Input: part model. Units: mm. Frame: model coordinates. A direction names the side the tool comes from. Give positions to 0.01 mm unless a question says otherwise; leave off trailing zeros. Loops run counter-clockwise (first coordinate to the right, second up) from the corner with the lowest first, then second, coordinate; pieces in that order, holes last. Notation, with made-up numbers: (63.5, -33.5) - (120.5, -33.5) arc R31 cw to (120.5, -4.5) - close; hole circle Ø3 at (64.5, 84). An arc over 180 degrees is marked (long way). One line per item, written item: value.
from build123d import *

# Parameters (mm, degrees)
F1_DEPTH = 63.5
F2_DEPTH = 25.4
F3_DEPTH = 7.9375
F0_W     = 25.4
F0_H     = 19.05
F4_DEPTH = 25.4
F6_R     = 5.08


# Not quite as in the source:
# - a feature names something its author has since deleted; it is built from what else it names


with BuildPart() as f1:
    # F0 (on Front) → F1 (new body, symmetric)
    with BuildSketch(Plane.XZ):
        Polygon((22.225, 9.525), (-41.275, 9.525), (-41.275, -9.525), (41.275, -9.525), (41.275, 9.525), align=None)
    extrude(amount=F1_DEPTH, both=True)

    # F0 (on Front) → F2 (join, symmetric)
    with BuildSketch(Plane.XZ):
        with BuildLine():
            Line((22.225, 27.0002), (22.225, 9.525))
            Line((22.225, 9.525), (41.275, 9.525))
            Line((41.275, 9.525), (41.275, 27.0002))
            ThreePointArc((41.275, 27.0002), (45.9246798487, 38.2255201513), (57.15, 42.8752))
            Line((57.15, 42.8752), (60.325, 42.8752))
            Line((60.325, 42.8752), (60.325, 61.9252))
            Line((60.325, 61.9252), (57.15, 61.9252))
            ThreePointArc((57.15, 61.9252), (32.4542956671, 51.6959043329), (22.225, 27.0002))
        make_face()
    extrude(amount=F2_DEPTH, both=True)

    # F0 (on Front) → F3 (join, symmetric)
    with BuildSketch(Plane.XZ):
        with BuildLine():
            add(Edge.make_bspline(
                [(-41.275, 9.525), (-39.190236479, 31.1887320131), (12.7593874931, 62.8514587879), (57.15, 61.9252)],
                knots=[0, 0, 0, 0, 111.5045361635, 111.5045361635, 111.5045361635, 111.5045361635], degree=3))
            Line((-41.275, 9.525), (22.225, 9.525))
            Line((22.225, 9.525), (22.225, 27.0002))
            ThreePointArc((22.225, 27.0002), (32.4542956671, 51.6959043329), (57.15, 61.9252))
        make_face()
    extrude(amount=F3_DEPTH, both=True)

    # F0 (on Front) → F4 (join, symmetric)
    with BuildSketch(Plane.XZ):
        with Locations((73.025, 52.4002)):
            Rectangle(F0_W, F0_H)
    extrude(amount=F4_DEPTH, both=True)

    # F0 (on Front) → F5 (revolve)
    with BuildSketch(Plane.XZ):
        Polygon((85.725, 66.675), (85.725, 61.9252), (85.725, 42.8752), (85.725, 38.1), (111.125, 38.1), (111.125, 66.675), align=None)
    revolve(axis=Axis((85.725, 0, 52.3875), (0, 0, -1)))

    # F6
    f6_edges = [f1.edges().sort_by_distance(p)[0] for p in [
        (41.275, -63.5, 0),
        (-41.275, -63.5, 0),
        (-41.275, 63.5, 0),
        (41.275, 63.5, 0),
    ]]
    fillet(f6_edges, radius=F6_R)


solid = f1.part
Item 1: Access query for faces 4 (the face through (46, -25.4, 42)), 5 (the face through (60, 2, 61.925)), 6 (the face through (45.8, -0.4, 38.1)). Directions: +Z, -Z, +X, -X, +Y, -Y. A direction counts if a zero-diameter tool reaches every point of the face in a straight line with its end or side. Return the directions, or none.
Verdict:
face 4: +Z, +X, -X, -Y
face 5: +Z, -X
face 6: -Z, +Y, -Y
Item 2: Material intervals for L1, parallel to Z at x = 68, y = -18 (3 decimals); L2, parallel to Z at x = -15.5, y = -38.5 (3 decimals); L3, parallel to X at y = -25.5, z = -4 (3 decimals), sorted ascending.
Verdict:
L1: z = 38.1 to 66.675
L2: z = -9.525 to 9.525
L3: x = -41.275 to 41.275
Item 3: Draft query along Y for faces 1 (the face through (1, -36, 9.525)), 2 (the face through (39.8, -62, 0.1)), 3 (the face through (46, 25.4, 42)). Return one class per face: pulls with the +Y half, pulls with the -Y half, needs draft (parallel to the pull), parting line crosses it, or undercut.
Verdict:
face 1: needs draft
face 2: pulls with the -Y half
face 3: pulls with the +Y half
Item 4: Pin query (flat end, axial travel): P1, Ø14, axis at y = 19.5, z = 20, coming from the -X side (3 decimals); P2, Ø8.5, axis at x = 67.5, y = -0.5, coming from the -Z side; P3, Ø4, axis at x = 45, y = -33.5, coming from the +Z side; P4, Ø1, axis at x = 1.5, z = 33, coming from the -Y side. Return the tip coordinate at first contact, or that it passes through.
Verdict:
P1: stops at x = 22.225
P2: stops at z = 38.1
P3: passes through
P4: stops at y = -7.94
Item 5: Section B-B, the plane y = 27.5. Output: boundary loops of the cut face in (x, z) (3 decimals).
Verdict:
outline: (-41.275, -9.525) - (41.275, -9.525) - (41.275, 9.525) - (-41.275, 9.525) - close
Item 6: Section A-A, the plane x = 64. Output: boundary loops of the cut face in (y, z) (3 decimals), and give its area (3 significant figures).
Verdict:
outline: (-25.4, 42.875) - (-13.16, 42.875) - (-13.16, 38.1) - (13.16, 38.1) - (13.16, 42.875) - (25.4, 42.875) - (25.4, 61.925) - (13.16, 61.925) - (13.16, 66.675) - (-13.16, 66.675) - (-13.16, 61.925) - (-25.4, 61.925) - close
area: 1,220 mm^2
Item 7: Section C-C, the plane x = 97. Output: boundary loops of the cut face in (y, z) (3 decimals).
Verdict:
outline: (-22.76, 38.1) - (22.76, 38.1) - (22.76, 66.675) - (-22.76, 66.675) - close
